Autodesk Fusion 360 part; units mm, degrees
sketch "Cigar Box" plane through (0, 0, 0) normal (0, 0, 1) x (1, 0, 0)
  line L0 (88.9, 36.875) -> (-88.9, 36.875)
  line L1 (-88.9, 36.875) -> (-88.9, -36.875)
  line L2 (-88.9, -36.875) -> (88.9, -36.875)
  line L3 (88.9, -36.875) -> (88.9, 36.875)
  line L4 (88.9, 36.875) -> (-88.9, -36.875) construction
  line L5 (-88.9, 36.875) -> (88.9, -36.875) construction
  line L6 (76.2, 24.175) -> (-76.2, 24.175)
  line L7 (-76.2, 24.175) -> (-76.2, 3.175)
  line L8 (-76.2, 3.175) -> (76.2, 3.175)
  line L9 (76.2, 3.175) -> (76.2, 24.175)
  line L10 (76.2, 24.175) -> (-76.2, 3.175) construction
  line L11 (-76.2, 24.175) -> (76.2, 3.175) construction
  line L12 (-76.2, 13.675) -> (76.2, 13.675)
  circle A0 centre (-63.5, 30.8) radius 4.075
  line L13 (-63.5, 30.8) -> (-63.5, 34.875) construction
  line L14 (-63.5, 34.875) -> (-63.5, 36.875) construction
  circle A1 centre (-63.5, -30.525) radius 3.375
  point P0 (0, 13.675)
  dimension "d1" = 177.8
  dimension "d3" = 152.4
  dimension "d4" = 21
  dimension "d5" = 3.175
  dimension "d6" = 8.15
  dimension "d7" = 2
  dimension "d8" = 25.4
  dimension "d9" = 12.7
  dimension "d10" = 6.75
  dimension "d11" = 6.35
  dimension "d12" = 25.4
extrude "Extrude1" add sketch "Cigar Box" against normal blind 24.13 contours L0 L1 L2 L3 | L6 L7 L9 L12 | L7 L8 L9 L12 | A0 | A1
extrude "Extrude2" cut sketch "Cigar Box" against normal blind 9 contours A0
extrude "Extrude3" cut sketch "Cigar Box" against normal blind 1.8 contours A1
mirror "Mirror1" about plane through (0, 0, 0) normal (1, 0, 0) of "Extrude3", "Extrude2"
revolve "Revolve1" cut sketch "Cigar Box" angle 360 about axis through (-76.2, 13.675, 0) along (1, 0, 0) contours L6 L7 L9 L12
mirror "Mirror2" about plane through (0, 0, 0) normal (0, 1, 0) of "Revolve1"
fillet "Fillet1" radius 6.35 4 edges at (88.9, -36.875, -12.065) (88.9, 36.875, -12.065) (-88.9, 36.875, -12.065) (-88.9, -36.875, -12.065)
fillet "Fillet1" radius 6.35 1 faces at (29.6333, -12.2917, -24.13)
For this review, take the finished solid that the model builds, in its own axes (mm). A direction names the side the tool comes from. Give positions to 0.01 mm unless a question says otherwise; leave off trailing zeros. Write each loop counter-clockwise with the first axis right and the second up, starting at its lowest first coordinate (ties: lowest second). Pieces come first, ordered by that corner, then holes. Notation, with made-up numbers: M -12.5,81.25 L 30.5,81.25 A17 ccw 30.5,108.25 Z; hole C -19.75,50 d10. An arc over 180 degrees is marked long. Answer as CSV lines item,"result".
1. Draft analysis for pull direction X (two halves, no side actions). For faces 1 (the flat face through (-1, 1, 0)), 2 (the cylindrical face through (86.99, 35.064, -9.014)), 3 (the cylindrical face through (-1.067, -13.444, -10.497)), state which applies: +X half, -X half, draft (parallel to the pull), parting line (faces both ways), or undercut.
Findings:
face 1,"draft"
face 2,"+X half"
face 3,"undercut"
2. Wall thickness on line 1 (Y direction, x = -63.5, z = -1.3) (3 decimals); line 2 (Y direction, x = -63.5, z = -4.5) (3 decimals); line 3 (X direction, y = -19, z = -6.5): over which ranges is each line inside the solid? List them lowest first.
Findings:
line 1,"y = -36.875 to -33.9, -27.15 to -24.094, -3.256 to 3.256, 24.094 to 26.725, 34.875 to 36.875"
line 2,"y = -36.875 to -23.162, -4.188 to 4.188, 23.162 to 26.725, 34.875 to 36.875"
line 3,"x = -88.9 to -76.2, 76.2 to 88.9"
3. For pin 1 (1 mm diameter, centred on x = 5.5, y = -21.5, fed in from +Z); pin 2 (10 mm diameter, centred on x = -2.5, y = 16, fed in from +Z); pin 3 (4 mm diameter, centred on x = -62.5, y = 30.5, fed in from +Z), all flat-tipped, find the tip position at first contact; note any pin that passes through.
Findings:
pin 1,"stops at z = -6.4"
pin 2,"stops at z = -7.52"
pin 3,"stops at z = -9"
4. Consider section B-B, the plane z = -4. Write out the cut boundary in (x, y) (3 decimals).
Findings:
outline,"M -88.9,-30.525 A6.35 ccw -82.55,-36.875 L 82.55,-36.875 A6.35 ccw 88.9,-30.525 L 88.9,30.525 A6.35 ccw 82.55,36.875 L -82.55,36.875 A6.35 ccw -88.9,30.525 Z; hole M -76.2,-23.383 L 76.2,-23.383 L 76.2,-3.967 L -76.2,-3.967 Z; hole M -76.2,3.967 L 76.2,3.967 L 76.2,23.383 L -76.2,23.383 Z; hole C -63.5,30.8 d8.15; hole C 63.5,30.8 d8.15"
5. Consider section C-C, the plane y = -7. Write out the cut boundary in (x, z), then the cut area to 3 significant figures.
Findings:
outline,"M -88.9,-17.78 A6.35 ccw -82.55,-24.13 L 82.55,-24.13 A6.35 ccw 88.9,-17.78 L 88.9,0 L 76.2,0 L 76.2,-8.11 L -76.2,-8.11 L -76.2,0 L -88.9,0 Z"
area,"3,040 mm2"
6. Consider section D-D, the plane x = 63.5. Write out the cut boundary in (y, z) (3 decimals), then the cut area to 3 significant figures.
Findings:
outline,"M -36.875,-17.78 A6.35 ccw -30.525,-24.13 L 30.525,-24.13 A6.35 ccw 36.875,-17.78 L 36.875,0 L 34.875,0 L 34.875,-9 L 26.725,-9 L 26.725,0 L 24.175,0 A10.5 cw 3.175,0 L -3.175,0 A10.5 cw -24.175,0 L -27.15,0 L -27.15,-1.8 L -33.9,-1.8 L -33.9,0 L -36.875,0 Z"
area,"1,330 mm2"
7. Consider section A-A, the plane x = 32. Write out the cut boundary in (y, z) (3 decimals).
Findings:
outline,"M -36.875,-17.78 A6.35 ccw -30.525,-24.13 L 30.525,-24.13 A6.35 ccw 36.875,-17.78 L 36.875,0 L 24.175,0 A10.5 cw 3.175,0 L -3.175,0 A10.5 cw -24.175,0 L -36.875,0 Z"
8. For faces 4 (the flat face through (-1, -36.875, -9)), 5 (the flat face through (-64, -30, -1.8)), list the 3-axis set-ups (+Z, -Z, +X, -X, +Y, -Y) from which the entire face can be reached by the end or side of a thin tool; tool diameter is ignored.
Findings:
face 4,"+Z, -Z, +X, -X, -Y"
face 5,"+Z"
